from build123d import *

# Parameters (mm, degrees)
F1_DEPTH = 20


with BuildPart() as f1:
    # F0 (on Front) → F1 (new body)
    with BuildSketch(Plane.XZ):
        with BuildLine():
            add(Edge.make_bspline(
                [(-21.722318, 57.734935), (-27.859297, 55.015494), (-32.833372, 51.301815), (-36.846273, 47.016584)],
                knots=[14.887886, 14.887886, 14.887886, 14.887886, 29.996616, 29.996616, 29.996616, 29.996616], degree=3))
            add(Edge.make_bspline(
                [(-36.846273, 47.016584), (-46.12578, 37.107336), (-50.265626, 24.14184), (-51.760266, 13.346677)],
                knots=[29.996616, 29.996616, 29.996616, 29.996616, 64.934324, 64.934324, 64.934324, 64.934324], degree=3))
            add(Edge.make_bspline(
                [(-51.760266, 13.346677), (-52.469743, 8.222425), (-52.583197, 3.587195), (-52.367426, 0)],
                knots=[64.934324, 64.934324, 64.934324, 64.934324, 81.518569, 81.518569, 81.518569, 81.518569], degree=3))
            add(Edge.make_bspline(
                [(-52.367426, 0), (-46.65998, -69.867425), (42.291667, -71.193181), (52.897733, 0)],
                knots=[0, 0, 0, 0, 105.265159, 105.265159, 105.265159, 105.265159], degree=3))
            add(Edge.make_bspline(
                [(52.210338, 14.565944), (52.768483, 9.85171), (52.974558, 4.967478), (52.897733, 0)],
                knots=[69.220725, 69.220725, 69.220725, 69.220725, 81.860246, 81.860246, 81.860246, 81.860246], degree=3))
            add(Edge.make_bspline(
                [(42.026516, 43.20865), (47.814994, 35.242619), (50.93367, 25.34899), (52.210338, 14.565944)],
                knots=[40.309872, 40.309872, 40.309872, 40.309872, 69.220725, 69.220725, 69.220725, 69.220725], degree=3))
            Line((42.026516, 43.20865), (42.026516, 36.341667))
            Line((42.026516, 36.341667), (42.005255, 43.237884))
            add(Edge.make_bspline(
                [(31.556576, 53.367701), (35.735048, 50.52724), (39.186175, 47.110795), (42.005255, 43.237884)],
                knots=[26.210335, 26.210335, 26.210335, 26.210335, 40.274494, 40.274494, 40.274494, 40.274494], degree=3))
            add(Edge.make_bspline(
                [(15.536849, 60.358789), (21.786503, 58.784782), (27.087548, 56.405678), (31.556576, 53.367701)],
                knots=[11.168201, 11.168201, 11.168201, 11.168201, 26.210335, 26.210335, 26.210335, 26.210335], degree=3))
            add(Edge.make_bspline(
                [(7.314677, 61.884856), (10.222105, 61.51986), (12.960106, 61.007755), (15.536849, 60.358789)],
                knots=[4.9663, 4.9663, 4.9663, 4.9663, 11.168201, 11.168201, 11.168201, 11.168201], degree=3))
            add(Edge.make_bspline(
                [(5.342527, 62.107149), (6.008411, 62.040455), (6.665764, 61.96632), (7.314677, 61.884856)],
                knots=[3.582089, 3.582089, 3.582089, 3.582089, 4.9663, 4.9663, 4.9663, 4.9663], degree=3))
            add(Edge.make_bspline(
                [(0, 62.473433), (1.839021, 62.402493), (3.619339, 62.27974), (5.342527, 62.107149)],
                knots=[0, 0, 0, 0, 3.582089, 3.582089, 3.582089, 3.582089], degree=3))
            add(Edge.make_bspline(
                [(0, 62.473433), (-1.86111, 62.397991), (-3.658814, 62.256857), (-5.395137, 62.05428)],
                knots=[0, 0, 0, 0, 3.260299, 3.260299, 3.260299, 3.260299], degree=3))
            Line((-5.395137, 62.05428), (-5.395137, 47.016584))
            Line((-5.395137, 47.016584), (-7.346095, 61.797247))
            add(Edge.make_bspline(
                [(-7.346095, 61.797247), (-12.036643, 61.107229), (-16.260302, 59.95632), (-20.060409, 58.435325)],
                knots=[4.497944, 4.497944, 4.497944, 4.497944, 13.546734, 13.546734, 13.546734, 13.546734], degree=3))
            add(Edge.make_bspline(
                [(-20.060409, 58.435325), (-20.623636, 58.209893), (-21.177558, 57.976331), (-21.722318, 57.734935)],
                knots=[13.546734, 13.546734, 13.546734, 13.546734, 14.887886, 14.887886, 14.887886, 14.887886], degree=3))
        make_face()
        with BuildLine():
            Line((-36.846273, 71.931325), (-36.846273, 47.016584))
            add(Edge.make_bspline(
                [(-21.722318, 57.734935), (-27.859297, 55.015494), (-32.833372, 51.301815), (-36.846273, 47.016584)],
                knots=[14.887886, 14.887886, 14.887886, 14.887886, 29.996616, 29.996616, 29.996616, 29.996616], degree=3))
            Line((-21.722318, 57.734935), (-21.722318, 71.931325))
            Line((-21.722318, 71.931325), (-21.722318, 78.35228))
            Line((-21.722318, 78.35228), (-36.846273, 78.35228))
            Line((-36.846273, 78.35228), (-36.846273, 71.931325))
        make_face()
        with BuildLine():
            add(Edge.make_bspline(
                [(-36.846273, 47.016584), (-46.12578, 37.107336), (-50.265626, 24.14184), (-51.760266, 13.346677)],
                knots=[29.996616, 29.996616, 29.996616, 29.996616, 64.934324, 64.934324, 64.934324, 64.934324], degree=3))
            Line((-36.846273, 47.016584), (-36.846273, 71.931325))
            Line((-36.846273, 71.931325), (-51.760266, 71.931325))
            Line((-51.760266, 71.931325), (-51.760266, 13.346677))
        make_face()
        with BuildLine():
            Line((-20.060409, 71.931325), (-20.060409, 58.435325))
            add(Edge.make_bspline(
                [(-7.346095, 61.797247), (-12.036643, 61.107229), (-16.260302, 59.95632), (-20.060409, 58.435325)],
                knots=[4.497944, 4.497944, 4.497944, 4.497944, 13.546734, 13.546734, 13.546734, 13.546734], degree=3))
            Line((-7.346095, 61.797247), (-8.683732, 71.931325))
            Line((-8.683732, 71.931325), (-20.060409, 71.931325))
        make_face()
        with BuildLine():
            add(Edge.make_bspline(
                [(-5.395137, 62.05428), (-6.054265, 61.977379), (-6.704547, 61.891624), (-7.346095, 61.797247)],
                knots=[3.260299, 3.260299, 3.260299, 3.260299, 4.497944, 4.497944, 4.497944, 4.497944], degree=3))
            Line((-7.346095, 61.797247), (-5.395137, 47.016584))
            Line((-5.395137, 47.016584), (-5.395137, 62.05428))
        make_face()
        with BuildLine():
            add(Edge.make_bspline(
                [(42.026516, 43.20865), (47.814994, 35.242619), (50.93367, 25.34899), (52.210338, 14.565944)],
                knots=[40.309872, 40.309872, 40.309872, 40.309872, 69.220725, 69.220725, 69.220725, 69.220725], degree=3))
            Line((52.210338, 14.565944), (52.210338, 85.566789))
            Line((52.210338, 85.566789), (42.026516, 85.566789))
            Line((42.026516, 85.566789), (42.026516, 43.20865))
        make_face()
        with BuildLine():
            Line((-5.395137, 71.931325), (-5.395137, 62.05428))
            add(Edge.make_bspline(
                [(0, 62.473433), (-1.86111, 62.397991), (-3.658814, 62.256857), (-5.395137, 62.05428)],
                knots=[0, 0, 0, 0, 3.260299, 3.260299, 3.260299, 3.260299], degree=3))
            add(Edge.make_bspline(
                [(0, 62.473433), (1.839021, 62.402493), (3.619339, 62.27974), (5.342527, 62.107149)],
                knots=[0, 0, 0, 0, 3.582089, 3.582089, 3.582089, 3.582089], degree=3))
            Line((5.342527, 62.107149), (5.230435, 75.449023))
            Line((5.230435, 75.449023), (5.206043, 78.35228))
            Line((5.206043, 78.35228), (-5.395137, 78.35228))
            Line((-5.395137, 78.35228), (-5.395137, 71.931325))
        make_face()
        with BuildLine():
            Line((42.026516, 36.341667), (42.026516, 43.20865))
            add(Edge.make_bspline(
                [(42.005255, 43.237884), (42.012346, 43.228142), (42.019433, 43.218397), (42.026516, 43.20865)],
                knots=[40.274494, 40.274494, 40.274494, 40.274494, 40.309872, 40.309872, 40.309872, 40.309872], degree=3))
            Line((42.005255, 43.237884), (42.026516, 36.341667))
        make_face()
        with BuildLine():
            add(Edge.make_bspline(
                [(31.556576, 53.367701), (35.735048, 50.52724), (39.186175, 47.110795), (42.005255, 43.237884)],
                knots=[26.210335, 26.210335, 26.210335, 26.210335, 40.274494, 40.274494, 40.274494, 40.274494], degree=3))
            Line((42.005255, 43.237884), (41.928474, 68.14196))
            Line((41.928474, 68.14196), (31.556576, 68.14196))
            Line((31.556576, 68.14196), (31.556576, 53.367701))
        make_face()
        with BuildLine():
            add(Edge.make_bspline(
                [(15.536849, 60.358789), (21.786503, 58.784782), (27.087548, 56.405678), (31.556576, 53.367701)],
                knots=[11.168201, 11.168201, 11.168201, 11.168201, 26.210335, 26.210335, 26.210335, 26.210335], degree=3))
            Line((31.556576, 53.367701), (31.556576, 68.14196))
            Line((31.556576, 68.14196), (31.556576, 78.35228))
            Line((31.556576, 78.35228), (17.436162, 78.35228))
            Line((17.436162, 78.35228), (15.536849, 60.358789))
        make_face()
        with BuildLine():
            Line((7.125281, 84.427975), (7.314677, 61.884856))
            add(Edge.make_bspline(
                [(7.314677, 61.884856), (10.222105, 61.51986), (12.960106, 61.007755), (15.536849, 60.358789)],
                knots=[4.9663, 4.9663, 4.9663, 4.9663, 11.168201, 11.168201, 11.168201, 11.168201], degree=3))
            Line((15.536849, 60.358789), (17.436162, 78.35228))
            Line((17.436162, 78.35228), (18.087206, 84.520072))
            Line((18.087206, 84.520072), (7.125281, 84.427975))
        make_face()
    extrude(amount=F1_DEPTH)


solid = f1.part
Design review of the part built by this model. Coordinates are the model's own, in mm. A direction names the side the tool comes from. Round coordinates to 2 decimals unless told otherwise and drop trailing zeros. Loops run counter-clockwise (first coordinate to the right, second up) from the corner with the lowest first, then second, coordinate; pieces in that order, holes last. Notation, with made-up numbers: (-37.75, -38) - (-8.75, -38) arc R18 cw to (-8.75, -6) - close; hole circle Ø4 at (-28, -36.5). An arc over 180 degrees is marked (long way). One line per item, written item: value. Start each with the question number.
1) For faces 1 (the flat face through (-8.006, -9.86, 66.793)), 2 (the flat face through (-1, -20, 26)), 3 (the flat face through (17.757, -9.86, 81.393)), 4 (the flat face through (-29, -10, 78.352)), list the 3-axis set-ups (+Z, -Z, +X, -X, +Y, -Y) from which the entire face can be reached by the end or side of a thin tool; tool diameter is ignored.
2) To check wall thickness, follow L1, parallel to X at y = -18.75, z = 69; L2, parallel to X at y = -5, z = 71.5; L3, parallel to X at y = -3, z = 76. State the ranges of each line that lie inside material, in increasing order. Write a range as from..to.
3) Draft analysis for pull direction X (two halves, no side actions). For faces 5 (the flat face through (31.557, -10, 73)), 6 (the flat face through (-1, 0, 26)), 7 (the flat face through (-36.846, -10, 75)), state which applies: +X half, -X half, draft (parallel to the pull), parting line (faces both ways), or undercut.
4) Consider section A-A on z = 60. Give the boundary of the cut face in (x, y).
5) Insertion check: pin 1 Ø3 at (x, y) = (-1.5, -10.5) entering from +Z; pin 2 Ø6 at (x, y) = (22.5, -16) entering from -Z; pin 3 Ø3 at (x, y) = (39.5, -10.5) entering from +Z. Each pin has a flat end and moves straight along its axis. Give the tip position at first contact, or say it passes through.
Reported:
1. face 1: +Z, +Y, -Y
1. face 2: +Z, -Z, +X, -X, -Y
1. face 3: +Y, -Y
1. face 4: +Z, -X, +Y, -Y
2. L1: x = -51.76..-21.72, -20.06..-8.3, -5.4..5.28, 7.25..31.56, 42.03..52.21
2. L2: x = -51.76..-21.72, -20.06..-8.63, -5.4..5.26, 7.23..31.56, 42.03..52.21
2. L3: x = -36.85..-21.72, -5.4..5.23, 7.2..31.56, 42.03..52.21
3. face 5: undercut
3. face 6: draft
3. face 7: -X half
4. outline: (-51.76, -20) - (-21.72, -20) - (-21.72, 0) - (-51.76, 0) - close; (-20.06, -20) - (41.95, -20) - (41.95, 0) - (-20.06, 0) - close; (42.03, -20) - (52.21, -20) - (52.21, 0) - (42.03, 0) - close
5. pin 1: stops at z = 78.35
5. pin 2: stops at z = -48.45
5. pin 3: stops at z = 68.14
